Here's how the part is built. I have some questions about the finished solid (model axes, mm). A direction names the side the tool comes from. Give positions to 0.01 mm unless a question says otherwise; leave off trailing zeros. Loops run counter-clockwise (first coordinate to the right, second up) from the corner with the lowest first, then second, coordinate; pieces in that order, holes last. Notation, with made-up numbers: M -5.75,-14 L 35.25,-14 A18 cw 35.25,2 Z; hole C -35,18 d1. An arc over 180 degrees is marked long. Answer as CSV lines item,"result". Start each with the question number.
Item 1: I want a section at B-B on x = 0. List the corners of the cut face in (y, z) for me (3 decimals), plus the area to 3 significant figures.
Item 2: I want a section at A-A on y = 0. List the corners of the cut face in (x, z) for me (3 decimals).
Item 3: For faces 5 (the cylindrical face through (-1.38, 6.2, 29.43)), 6 (the cylindrical face through (5.45, -1.72, 31.31)), which set-ups out of +Z, -Z, +X, -X, +Y, -Y let a thin tool reach every point of the face, with its end or its side?
Item 4: I want a section at C-C on x = -4.5. List the corners of the cut face in (y, z) for me.
Item 5: I want a section at D-D on z = 5.08. List the corners of the cut face in (x, y) for me (3 decimals), plus the area to 3 significant figures.
Item 6: If I drill on line 1 along Z through (x, y) = (0, -6.1); line 2 along Z through (x, y) = (-5.5, -6.25); line 3 along Y through (x, z) = (2, 10.5), over which ranges is the centre line in solid material (lowest first)? Write a range as from..to.
Item 7: If we mould it in two halves opening along X, with no side actions, what happens to faces 1 (the cylindrical face through (1.37, -5.73, 2.94)), 2 (the cylindrical face through (-2.016, 5.743, 6.626)), 3 (the flat face through (-6, 1, 0)), 4 (the cylindrical face through (-7.559, -5.796, 61.622))? For each: released by +X, released by -X, zero draft, split by the parting line, or undercut.
Item 8: Will these pins go through, and if not, where does the flat tip stop? P1, Ø4, axis at x = 2.5, z = 51, coming from the +Y side; P2, Ø10, axis at x = -3, z = 32.5, coming from the -Y side; P3, Ø1.5, axis at x = 4, z = 52.5, coming from the -Y side.
Autodesk Inventor part; units mm, degrees
ref_plane "Work Plane2" through (0, 6.35, 0) normal (0, 1, 0) x (1, 0, 0)
ref_plane "YZ Plane" through (0, 0, 0) normal (1, 0, 0) x (0, 1, 0)
ref_plane "XZ Plane" through (0, 0, 0) normal (0, 1, 0) x (-1, 0, 0)
sketch "Sketch1" plane through (0, 0, 0) normal (0, 0, 1) x (1, 0, 0)
  circle A0 centre (0, 0) radius 6.35
  circle A1 centre (0, 0) radius 5.715
  dimension "d0" = 12.7
  dimension "d1" = 11.43
extrude "Extrusion1" add sketch "Sketch1" along normal blind 63.5
sketch "Sketch2" plane through (0, 0, 63.5) normal (0, 0, 1) x (1, 0, 0)
  circle A0 centre (0, 0) radius 6.35
  circle A1 centre (0, 0) radius 9.525
  dimension "d4" = 19.05
extrude "Extrusion2" add sketch "Sketch2" against normal blind 3.81
sketch "Sketch3" plane through (0, 0, 0) normal (0, 0, -1) x (-1, 0, 0)
  circle A0 centre (0, 0) radius 5.715
  circle A1 centre (0, 0) radius 6.35
  line L0 (0, 0) -> (-6.35, 0)
ref_plane "Work Plane2" through (0, 6.35, 0) normal (0, 1, 0) x (1, 0, 0)
ref_plane "Work Plane1" through (0, 0, 0) normal (0, 1, 0) x (1, 0, 0)
sketch "Sketch4" plane through (0, 6.35, 0) normal (0, 1, 0) x (1, 0, 0)
  line L0 (0, 0) -> (0, -5.08)
  circle A0 centre (0, -5.08) radius 2.54
  dimension "d9" = 5.08
  dimension "d10" = 5.08
extrude "Extrusion3" cut sketch "Sketch4" against normal blind 50.8
properties part number "LongPin" material "Steel"
Result:
1,outline,"M -9.525,59.69 L -6.35,59.69 L -6.35,7.62 L -5.715,7.62 L -5.715,63.5 L -9.525,63.5 Z; M -6.35,0 L -5.715,0 L -5.715,2.54 L -6.35,2.54 Z; M 5.715,0 L 6.35,0 L 6.35,2.54 L 5.715,2.54 Z; M 5.715,7.62 L 6.35,7.62 L 6.35,59.69 L 9.525,59.69 L 9.525,63.5 L 5.715,63.5 Z"
1,area,"98.4 mm^2"
2,outline,"M -9.525,59.69 L -6.35,59.69 L -6.35,0 L -5.715,0 L -5.715,63.5 L -9.525,63.5 Z; M 5.715,0 L 6.35,0 L 6.35,59.69 L 9.525,59.69 L 9.525,63.5 L 5.715,63.5 Z"
3,face 5,"-Z"
3,face 6,"+Z, -Z"
4,outline,"M -8.39,59.69 L -4.48,59.69 L -4.48,0 L -3.52,0 L -3.52,63.5 L -8.39,63.5 Z; M 3.52,0 L 4.48,0 L 4.48,59.69 L 8.39,59.69 L 8.39,63.5 L 3.52,63.5 Z"
5,outline,"M -2.54,-5.82 L -2.54,-5.12 A5.715 cw -2.54,5.12 L -2.54,5.82 A6.35 ccw Z; M 2.54,-5.82 A6.35 ccw 2.54,5.82 L 2.54,5.12 A5.715 cw 2.54,-5.12 Z"
5,area,"17.4 mm^2"
6,line 1,"0..2.54, 7.62..63.5"
6,line 2,"59.69..63.5"
6,line 3,"-6.03..-5.35, 5.35..6.03"
7,face 1,"undercut"
7,face 2,"undercut"
7,face 3,"zero draft"
7,face 4,"split by the parting line"
8,P1,"y = 6.33"
8,P2,"y = -6.35"
8,P3,"y = -5.46"
